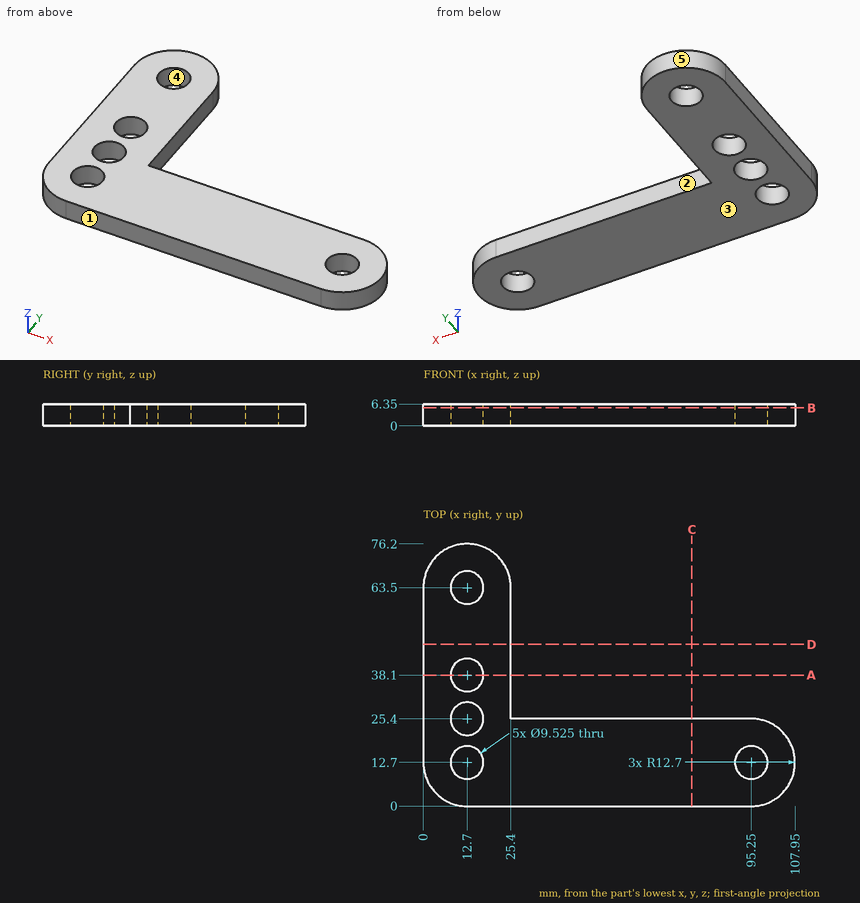
Job drawing, mm, ordinate dimensions from the low corner. One solid piece. A direction names the side the tool comes from. Round coordinates to 2 decimals unless told otherwise and drop trailing zeros. Order: outer loops, then holes, each group sorted by start corner. A loop starts at its lowest first (then second) coordinate and runs counter-clockwise, first axis right, second up. Notation, with made-up numbers: (-20, -22) - (12, -22) arc R13 cw to (12, -5) - close; hole circle Ø4 at (72.25, 62). An arc over 180 degrees is marked (long way). Use CSV: the item, a comma, the result in double quotes. Start each with the question number.
1) Saw through at B-B (z = 5.25). Count the separate pieces of the cut face and the enclosed holes in it, and give its area (3 significant figures).
2) Wall check: L1, parallel to Y at x = 15, z = 6.25; L2, parallel to X at y = 38, z = 5.5; L3, parallel to Y at x = 91.5, z = 1.75. Give the ranges that are in metal, low to high. Write a range as [from, to].
3) Saw through at A-A (y = 38.1). List the corners of the cut face in (x, z).
4) Pin check, flat tips, straight feed: pin 1 Ø1.5 at (x, z) = (16, 5.5) entering from +Y; pin 2 Ø2 at (y, z) = (53.5, 5) entering from +X. Stop position of each tip, or through.
5) Two-plate mould, pull along X, no slides. Class the marked faces 3, 4 and 5: pulls with the +X half, pulls with the -X half, needs draft (parallel to the pull), parting line crosses it, or undercut.
6) Saw through at C-C (x = 78). List the corners of the cut face in (y, z), and give its area (3 significant figures).
7) Tool access for the marked faces 1 and 2: list every direction of +Z, -Z, +X, -X, +Y, -Y with a clear straight run to the whole face (end or side of a thin tool).
Values follow:
1,separate pieces,"1"
1,enclosed holes,"5"
1,area,"3,500 mm2"
2,L1,"y = [0, 8.53], [16.87, 21.23], [29.57, 33.93], [42.27, 59.33], [67.67, 75.99]"
2,L2,"x = [0, 7.94], [17.46, 25.4]"
2,L3,"y = [0, 9.76], [15.64, 25.4]"
3,outline,"(0, 0) - (7.94, 0) - (7.94, 6.35) - (0, 6.35) - close; (17.46, 0) - (25.4, 0) - (25.4, 6.35) - (17.46, 6.35) - close"
4,pin 1,"stops at y = 75.94"
4,pin 2,"stops at x = 25.4"
5,face 3,"needs draft"
5,face 4,"undercut"
5,face 5,"parting line crosses it"
6,outline,"(0, 0) - (25.4, 0) - (25.4, 6.35) - (0, 6.35) - close"
6,area,"161 mm2"
7,face 1,"+Z, -Z, +X, -X, -Y"
7,face 2,"+Z, -Z, +X, +Y"
